```python
from build123d import *

# Parameters (mm, degrees)
SKETCH1_R           = 1.5
BOSS_EXTRUDE1_DEPTH = 3


with BuildPart() as part:
    # Sketch1 → Boss-Extrude1 (new body)
    with BuildSketch(Plane.XY):
        with BuildLine():
            Line((50, -5), (-50, -5))
            Line((-50, -5), (-55, -5))
            Line((-55, -5), (-55, 0))
            ThreePointArc((-55, 0), (-53.535533906, 3.535533906), (-50, 5))
            Line((-50, 5), (50, 5))
            ThreePointArc((50, 5), (53.535533906, 3.535533906), (55, 0))
            Line((55, 0), (55, -5))
            Line((55, -5), (50, -5))
        make_face()
        with Locations((50, 0)):
            Circle(SKETCH1_R, mode=Mode.SUBTRACT)
        with BuildLine():
            Line((-50, 1.5), (-30, 1.5))
            ThreePointArc((-30, 1.5), (-28.5, 0), (-30, -1.5))
            Line((-30, -1.5), (-50, -1.5))
            ThreePointArc((-50, -1.5), (-51.5, 0), (-50, 1.5))
        make_face(mode=Mode.SUBTRACT)
    extrude(amount=BOSS_EXTRUDE1_DEPTH)


solid = part.part
```
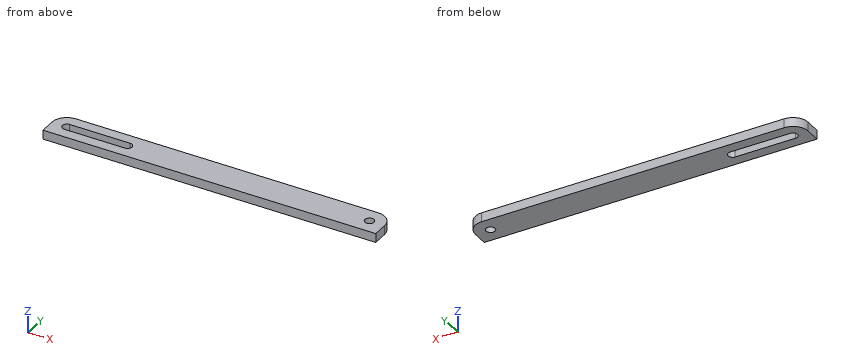
The model under review builds one solid part; all positions refer to its coordinate system, in mm. Round coordinates to 2 decimals unless told otherwise and drop trailing zeros. Order: outer loops, then holes, each group sorted by start corner. A loop starts at its lowest first (then second) coordinate and runs counter-clockwise, first axis right, second up. Notation, with made-up numbers: (78, -30) -> (94, -30) arc R28 cw to (94, 8) -> close; hole circle Ø10 at (3, 66.25). An arc over 180 degrees is marked (long way). One line per item, written item: value. Start each with the question number.
Q1. Take a section at A-A (z = 0.7). Write out the cut boundary in (x, y).
Q2. Wall thickness on line 1 (Y direction, x = 50, z = 1.85); line 2 (X direction, y = -0.5, z = 0.75); line 3 (X direction, y = 1, z = 2.5): over which ranges is each line inside the solid? List them lowest first.
Q3. Clearance check with a flat-ended pin moving along its axis: pin 1 Ø3.5 at (x, y) = (50, 0) entering from -Z. State where the tip first meets the part, or that it passes through.
Reported:
1. outline: (-55, -5) -> (55, -5) -> (55, 0) arc R5 ccw to (50, 5) -> (-50, 5) arc R5 ccw to (-55, 0) -> close; hole (-50, -1.5) -> (-30, -1.5) arc R1.5 ccw to (-30, 1.5) -> (-50, 1.5) arc R1.5 ccw to start; hole circle Ø3 at (50, 0)
2. line 1: y = -5 to -1.5, 1.5 to 5
2. line 2: x = -55 to -51.41, -28.59 to 48.59, 51.41 to 55
2. line 3: x = -54.9 to -51.12, -28.88 to 48.88, 51.12 to 54.9
3. pin 1: stops at z = 0
